from build123d import *

# Parameters (mm, degrees)
EXTRUDE_1_DEPTH = 60
EXTRUDE_START   = 5
SKETCH_2_R      = 1.5
EXTRUDE_2_DEPTH = 5
CHAMFER_1_SIZE  = 5


with BuildPart() as part:
    # 草图1 → 凸台-拉伸1 (new body)
    with BuildSketch(Plane.XY):
        with BuildLine():
            Line((0, 112.5), (0, 115.5))
            ThreePointArc((0, 115.5), (23.613333333, 113.060428484), (46.22915298, 105.84477037))
            Line((46.22915298, 105.84477037), (45.02839576, 103.095555556))
            ThreePointArc((45.02839576, 103.095555556), (23, 110.123793978), (0, 112.5))
        make_face()
    extrude(amount=EXTRUDE_1_DEPTH)

    # 草图2 → 凸台-拉伸2 (add)
    with BuildSketch(Plane(origin=(0, 0, 35), x_dir=(-1, 0, 0), z_dir=(0, 0, -1)).offset(EXTRUDE_START)):
        with BuildLine():
            Line((-27.702222222, 132.637991857), (-4.587645732, 137.465606672))
            Line((-4.587645732, 137.465606672), (0, 115.5))
            ThreePointArc((0, 115.5), (-23.613333333, 113.060428484), (-46.22915298, 105.84477037))
            Line((-46.22915298, 105.84477037), (-50.816798712, 127.810377043))
            Line((-50.816798712, 127.810377043), (-27.702222222, 132.637991857))
        make_face()
        with Locations((-8.570753879, 131.525823236)):
            Circle(SKETCH_2_R, mode=Mode.SUBTRACT)
        with Locations(Location((-44.789246121, 123.961378792, 0), (0, 0, 180))):
            Circle(SKETCH_2_R, mode=Mode.SUBTRACT)
    extrude(amount=-EXTRUDE_2_DEPTH)

    # 倒角1
    chamfer_1_edges = [part.edges().sort_by_distance(p)[0] for p in [
        (23.613333333, 113.060428484, 35),
    ]]
    chamfer(chamfer_1_edges, length=CHAMFER_1_SIZE)


solid = part.part
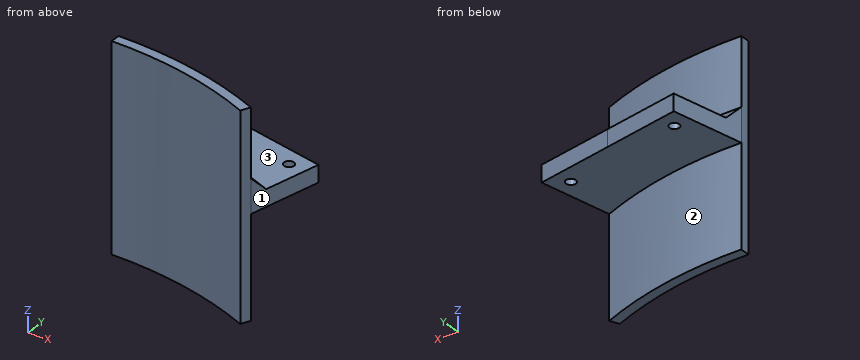
The model under review builds one solid part; all positions refer to its coordinate system, in mm. Face numbers are marked on the shaded views. A direction names the side the tool comes from. Coordinates: 2 decimals unless noted, no trailing zeros. Loops run counter-clockwise (first coordinate to the right, second up) from the corner with the lowest first, then second, coordinate; pieces in that order, holes last.
(1) Insertion check: P1, Ø5, axis at x = 37, z = 7.5, coming from the -Y side; P2, Ø12, axis at y = 111, z = 30, coming from the +X side; P3, Ø5, axis at x = 36, z = 25.5, coming from the -Y side. Each pin has a flat end and moves straight along its axis. Give the tip position at first contact, or say it passes through.
Determined:
P1: stops at y = 105.34
P2: stops at x = 48.56
P3: stops at y = 105.71
(2) Tool access review of the marked faces 1, 2 and 3: name each direction out of +Z, -Z, +X, -X, +Y, -Y from which nothing blocks a thin tool from reaching the whole face with its end or side.
Determined:
face 1: +Z, -Z, +X, -Y
face 2: -Z, +X, +Y
face 3: +Z, +X, +Y
(3) Consider section B-B, the plane y = 129. Give the boundary of the cut face in (x, z), plus the area to 3 significant figures.
Determined:
outline: (2.82, 30) - (45.12, 30) - (45.12, 35) - (2.82, 35) - close
area: 212 mm2
(4) Consider section A-A, the plane z = 43.5. Give the boundary of the cut face in (x, y), plus the area to 3 significant figures.
Determined:
outline: (0, 112.5) arc R112.5 cw to (45.03, 103.1) - (46.23, 105.84) arc R115.5 ccw to (0, 115.5) - close
area: 141 mm2
(5) Wall thickness on L1, parallel to Z at x = 13, y = 135; L2, parallel to Y at x = 18, z = 39.5; L3, parallel to Y at x = 32, z = 39.5: over which ranges is each line inside the solid? List them lowest first.
Determined:
L1: z = 30 to 35
L2: y = 111.05 to 114.59
L3: y = 107.85 to 111.5
